Here's how the part is built. I have some questions about the finished solid (model axes, mm). Coordinates: 2 decimals unless noted, no trailing zeros. Write each loop counter-clockwise with the first axis right and the second up, starting at its lowest first coordinate (ties: lowest second). Pieces come first, ordered by that corner, then holes.
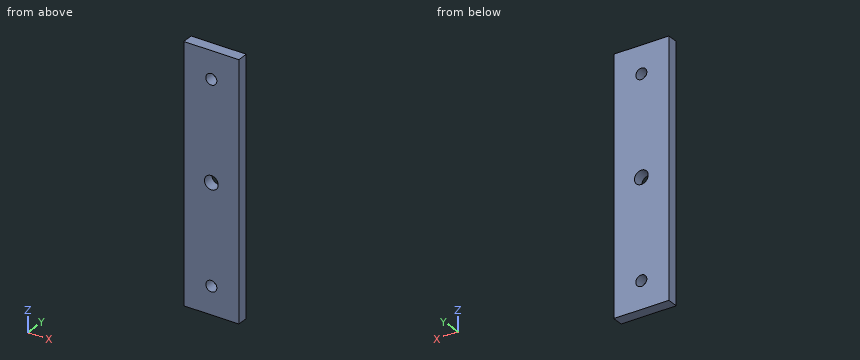
```python
from build123d import *

# Parameters (mm, degrees)
SKETCH1_W           = 100
SKETCH1_H           = 460
SKETCH1_R           = 10
BOSS_EXTRUDE1_DEPTH = 20
SKETCH2_R           = 12.5
CUT_EXTRUDE1_DEPTH  = 21


with BuildPart() as part:
    # Sketch1 → Boss-Extrude1 (new body)
    with BuildSketch(Plane(origin=(0, 0, 0), x_dir=(1, 0, 0), z_dir=(0, 1, 0))):
        Rectangle(SKETCH1_W, SKETCH1_H)
        with Locations((0, -180)):
            Circle(SKETCH1_R, mode=Mode.SUBTRACT)
        with Locations((0, 180)):
            Circle(SKETCH1_R, mode=Mode.SUBTRACT)
    extrude(amount=BOSS_EXTRUDE1_DEPTH)

    # Sketch2 → Cut-Extrude1 (cut, through all)
    with BuildSketch(Plane(origin=(0, 20, 0), x_dir=(1, 0, 0), z_dir=(0, 1, 0))):
        Circle(SKETCH2_R)
    extrude(amount=-CUT_EXTRUDE1_DEPTH, mode=Mode.SUBTRACT)


solid = part.part
```
1) I need wall thicknesses on probe 1 along Z at (x, y) = (0, 11); probe 2 along X at (y, z) = (9.25, 0); probe 3 along X at (y, z) = (15.25, -180). Which ranges of each line are inside material? Lowest first, please.
Values follow:
probe 1: z = -230 to -190, -170 to -12.5, 12.5 to 170, 190 to 230
probe 2: x = -50 to -12.5, 12.5 to 50
probe 3: x = -50 to -10, 10 to 50
2) Imagine slicing it at B-B on z = 0. Please give me the cut outline in (x, y), then the cut area to 3 significant figures.
Values follow:
outline: (-50, 0) - (-12.5, 0) - (-12.5, 20) - (-50, 20) - close; (12.5, 0) - (50, 0) - (50, 20) - (12.5, 20) - close
area: 1,500 mm2
3) Imagine slicing it at D-D on z = -180. Please give me the cut outline in (x, y).
Values follow:
outline: (-50, 0) - (-10, 0) - (-10, 20) - (-50, 20) - close; (10, 0) - (50, 0) - (50, 20) - (10, 20) - close
4) Imagine slicing it at C-C on y = 14. Please give me the cut outline in (x, z), then the cut area to 3 significant figures.
Values follow:
outline: (-50, -230) - (50, -230) - (50, 230) - (-50, 230) - close; hole circle Ø25 at (0, 0); hole circle Ø20 at (0, -180); hole circle Ø20 at (0, 180)
area: 44,900 mm2
5) Imagine slicing it at A-A on x = 0. Please give me the cut outline in (y, z).
Values follow:
outline: (0, -230) - (20, -230) - (20, -190) - (0, -190) - close; (0, -170) - (20, -170) - (20, -12.5) - (0, -12.5) - close; (0, 12.5) - (20, 12.5) - (20, 170) - (0, 170) - close; (0, 190) - (20, 190) - (20, 230) - (0, 230) - close
6) Will this pin go through, and if not, where does the flat tip stop? pin 1 (12 mm diameter, centred on x = 0, z = -180, fed in from -Y).
Values follow:
pin 1: passes through
